Source: CAD feature listing. Evaluate the final solid. Frame: model axes, mm. Face numbers are marked on the shaded views. A direction names the side the tool comes from. Coordinates: 2 decimals unless noted, no trailing zeros. Order: outer loops, then holes, each group sorted by start corner. A loop starts at its lowest first (then second) coordinate and runs counter-clockwise, first axis right, second up.
Item 1: Section C-C on y = 3. Return the cut outline in (x, z), then the cut area to 3 significant figures.
Item 2: Ray query, line 1 (Y direction, x = -16, z = 4.5); line 2 (Y direction, x = -31, z = 4.5); line 3 (Y direction, x = 11, z = 3.5). Return the intervals inside material, ascending.
Item 3: Section B-B on z = 5.25. Return the cut outline in (x, y).
Item 4: Contact query for flat-ended pins moving along their axis: P1, Ø1, axis at x = -3.5, z = 4.5, coming from the +Y side; P2, Ø1.5, axis at y = 8.5, z = 3, coming from the -X side; P3, Ø3, axis at x = 31, y = 0, coming from the -Z side; P4, Ø1, axis at x = 8, y = 0, coming from the +Z side. Output: stop coordinate, or through.
Item 5: Section D-D on y = -0.75. Return the cut outline in (x, z).
Item 6: Reachability of the marked faces 1, 2 and 3 from +Z, -Z, +X, -X, +Y, -Y: full face, straight path, thin tool, end or side. Return the list, or none.
Item 7: Mould query, pull axis Y, two halves, no side actions, for the marked faces 4, 5 and 6. Classes: released by +Y, released by -Y, zero draft, split by the parting line, or undercut.
Item 8: Section A-A on x = 0. Return the cut outline in (y, z).
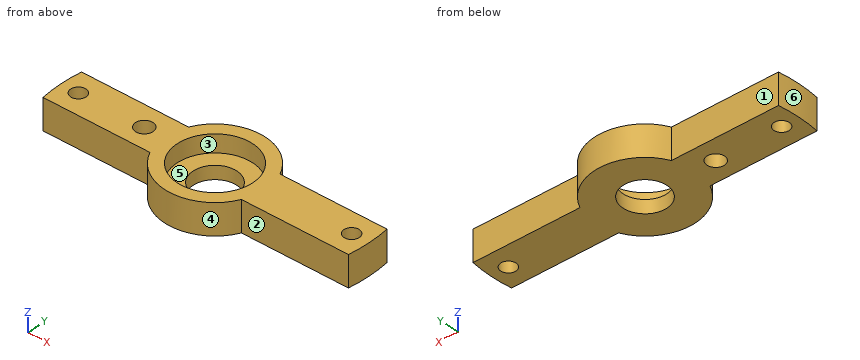
Autodesk Fusion 360 part; units mm, degrees
sketch "Szkic1" plane through (0, 0, 0) normal (0, 0, 1) x (1, 0, 0)
  circle A0 centre (0, 0) radius 11.5
  circle A1 centre (0, 0) radius 8.6
  circle A2 centre (0, 0) radius 5
  dimension "d1" = 23
  dimension "d2" = 17.2
  dimension "d7" = 10
extrude "Wyciągnięcie proste1" add sketch "Szkic1" along normal blind 7 contours A0
extrude "Wyciągnięcie proste2" add sketch "Szkic1" along normal blind 3 contours A1
sketch "Szkic2" plane through (0, 0, 0) normal (0, 0, 1) x (1, 0, 0)
  line L0 (20, -5) -> (-20, -5)
  line L1 (-20, 5) -> (20, 5)
  line L2 (20, -5) -> (-20, 5) construction
  line L3 (-20, -5) -> (20, 5) construction
  line L4 (35, -4.95) -> (-35, -4.95)
  line L5 (-35, -4.95) -> (-35, 4.95)
  line L6 (-35, 4.95) -> (35, 4.95)
  line L7 (35, 4.95) -> (35, -4.95)
  line L8 (35, -4.95) -> (-35, 4.95) construction
  line L9 (-20, -5) -> (-24, -5)
  line L10 (-24, 5) -> (-20, 5)
  circle A0 centre (0, 0) radius 11.5
  line L11 (-35, -4.95) -> (-11.3867, -1.6104) construction
  line L12 (0, 0) -> (35, 4.95) construction
  circle A1 centre (0, 0) radius 35
  circle A2 centre (-31, 0) radius 1.75
  circle A3 centre (31, 0) radius 1.75
  circle A4 centre (-15.9999, -0.05) radius 2
  dimension "d9" = 10
  dimension "d10" = 70
  dimension "d11" = 9.9
  dimension "d36" = 3.5
  dimension "d37" = 4
  dimension "d38" = 4
  dimension "d68" = 4
  dimension "d69" = 5
  dimension "d70" = 16
extrude "Wyciągnięcie proste3" add sketch "Szkic2" along normal blind 7 contours L4 L6 A0 A1 | L4 L6 A0 A1
Answer list:
1. outline: (-34.87, 0) - (-4, 0) - (-4, 3) - (-8.06, 3) - (-8.06, 7) - (-34.87, 7) - close; (4, 0) - (34.87, 0) - (34.87, 7) - (8.06, 7) - (8.06, 3) - (4, 3) - close
1. area: 400 mm2
2. line 1: y = -4.95 to -2.05, 1.95 to 4.95
2. line 2: y = -4.95 to -1.75, 1.75 to 4.95
2. line 3: y = -4.95 to 4.95
3. outline: (-34.65, -4.95) - (-10.38, -4.95) arc R11.5 ccw to (10.38, -4.95) - (34.65, -4.95) arc R35 ccw to (34.65, 4.95) - (10.38, 4.95) arc R11.5 ccw to (-10.38, 4.95) - (-34.65, 4.95) arc R35 ccw to start; hole circle Ø3.5 at (-31, 0); hole circle Ø4 at (-16, -0.05); hole circle Ø17.2 at (0, 0); hole circle Ø3.5 at (31, 0)
4. P1: stops at y = 11.1
4. P2: stops at x = -8.5
4. P3: passes through
4. P4: stops at z = 3
5. outline: (-34.99, 0) - (-32.58, 0) - (-32.58, 7) - (-34.99, 7) - close; (-29.42, 0) - (-17.87, 0) - (-17.87, 7) - (-29.42, 7) - close; (-14.13, 0) - (-4.94, 0) - (-4.94, 3) - (-8.57, 3) - (-8.57, 7) - (-14.13, 7) - close; (4.94, 0) - (29.42, 0) - (29.42, 7) - (8.57, 7) - (8.57, 3) - (4.94, 3) - close; (32.58, 0) - (34.99, 0) - (34.99, 7) - (32.58, 7) - close
6. face 1: +Z, -Z, -X, +Y
6. face 2: +Z, -Z, +X, -Y
6. face 3: +Z
7. face 4: released by -Y
7. face 5: undercut
7. face 6: split by the parting line
8. outline: (-11.5, 0) - (-5, 0) - (-5, 3) - (-8.6, 3) - (-8.6, 7) - (-11.5, 7) - close; (5, 0) - (11.5, 0) - (11.5, 7) - (8.6, 7) - (8.6, 3) - (5, 3) - close
